Autodesk Inventor part; units mm, degrees
ref_plane "YZ Plane" through (0, 0, 0) normal (1, 0, 0) x (0, 1, 0)
ref_plane "XZ Plane" through (0, 0, 0) normal (0, 1, 0) x (-1, 0, 0)
ref_plane "XY Plane" through (0, 0, 0) normal (0, 0, 1) x (1, 0, 0)
sketch "Sketch1" plane through (0, 0, 0) normal (0, 1, 0) x (-1, 0, 0)
  line L0 (0, 0) -> (48.65, 0)
  line L1 (48.65, 0) -> (48.65, -41.19)
  line L2 (48.65, -41.19) -> (0, -41.19)
  line L3 (0, -41.19) -> (0, 0)
  dimension "d0" = 48.65
  dimension "d1" = 41.19
extrude "Extrusion1" add sketch "Sketch1" along normal blind 1
sketch "Sketch2" plane through (0, 1, 0) normal (0, 1, 0) x (1, 0, 0)
  line L0 (0, 0) -> (-18.8, 0)
  line L1 (-48.65, 0) -> (0, 0)
  line L2 (-18.8, 0) -> (-18.8, 8.64)
  line L3 (0, 0) -> (-33.02, 0)
  line L4 (-30.48, 20.32) -> (-30.48, 21.59)
  line L5 (-30.48, 16.51) -> (-30.48, 13.97)
  line L6 (0, 41.19) -> (-48.65, 41.19)
  line L7 (0, 0) -> (0, 41.19)
  line L8 (-48.65, 41.19) -> (-48.65, 0)
  point P0 (-18.8, 11.18)
  point P1 (-18.8, 13.72)
  point P2 (-18.8, 16.26)
  point P3 (-18.8, 18.8)
  point P4 (-18.8, 21.34)
  point P5 (-18.8, 23.88)
  point P6 (-18.8, 26.42)
  point P7 (-18.8, 28.96)
  point P8 (-18.8, 31.5)
  point P9 (-21.34, 8.64)
  point P10 (-21.34, 11.18)
  point P11 (-21.34, 13.72)
  point P12 (-21.34, 16.26)
  point P13 (-21.34, 18.8)
  point P14 (-21.34, 21.34)
  point P15 (-21.34, 23.88)
  point P16 (-21.34, 26.42)
  point P17 (-21.34, 28.96)
  point P18 (-21.34, 31.5)
  point P19 (-30.48, 24.13)
  point P20 (-46.74, 8.64)
  point P21 (-46.74, 8.64)
  point P22 (-46.74, 11.18)
  point P23 (-46.74, 13.72)
  point P24 (-46.74, 16.26)
  point P25 (-46.74, 18.8)
  point P26 (-46.74, 21.34)
  point P27 (-46.74, 23.88)
  point P28 (-46.74, 26.42)
  point P29 (-46.74, 28.96)
  point P30 (-46.74, 31.5)
  point P31 (-44.2, 8.64)
  point P32 (-44.2, 11.18)
  point P33 (-44.2, 13.72)
  point P34 (-44.2, 16.26)
  point P35 (-44.2, 18.8)
  point P36 (-44.2, 21.34)
  point P37 (-44.2, 23.88)
  point P38 (-44.2, 26.42)
  point P39 (-44.2, 28.96)
  point P40 (-44.2, 31.5)
  point P41 (-30.48, 19.05)
  point P42 (-30.48, 19.05)
  point P43 (-30.48, 24.13)
  point P44 (-30.48, 26.67)
  dimension "d4" = 18.8
  dimension "d5" = 8.64
  dimension "d8" = 2.54
  dimension "d11" = 2.54
  dimension "d14" = 33.02
  dimension "d19" = 2.54
  dimension "d26" = 2.54
  dimension "d77" = 41.19
  dimension "d78" = 48.641
  dimension "d89" = 30.48
hole "Hole1" at (-18.8, 1, -8.64) at (-18.8, 1, -11.18) at (-18.8, 1, -13.72) at (-18.8, 1, -16.26) at (-18.8, 1, -18.8) at (-18.8, 1, -21.34) at (-18.8, 1, -23.88) at (-18.8, 1, -26.42) at (-18.8, 1, -28.96) at (-18.8, 1, -31.5) at (-21.34, 1, -8.64) at (-21.34, 1, -11.18) at (-21.34, 1, -13.72) at (-21.34, 1, -16.26) at (-21.34, 1, -18.8) at (-21.34, 1, -21.34) at (-21.34, 1, -23.88) at (-21.34, 1, -26.42) at (-21.34, 1, -28.96) at (-21.34, 1, -31.5) at (-30.48, 1, -21.59) at (-30.48, 1, -24.13) at (-30.48, 1, -16.51) at (-44.2, 1, -31.5) at (-44.2, 1, -28.96) at (-44.2, 1, -26.42) at (-44.2, 1, -23.88) at (-44.2, 1, -21.34) at (-44.2, 1, -18.8) at (-44.2, 1, -16.26) at (-44.2, 1, -13.72) at (-44.2, 1, -11.18) at (-44.2, 1, -8.64) at (-46.74, 1, -31.5) at (-46.74, 1, -28.96) at (-46.74, 1, -26.42) at (-46.74, 1, -23.88) at (-46.74, 1, -21.34) at (-46.74, 1, -18.8) at (-46.74, 1, -16.26) at (-46.74, 1, -13.72) at (-46.74, 1, -11.18) at (-46.74, 1, -8.64) at (-30.48, 1, -19.05) at (-30.48, 1, -26.67) at (-30.48, 1, -13.97) direction (0, -1, 0) diameter 1.5 end through all
sketch "Sketch3" plane through (0, 1, 0) normal (0, 1, 0) x (1, 0, 0)
  line L0 (-28.956, 38.735) -> (-26.924, 38.735)
  line L1 (-26.924, 38.735) -> (-26.924, 37.465)
  line L2 (-26.924, 37.465) -> (-28.956, 37.465)
  line L3 (-28.956, 37.465) -> (-28.956, 38.735)
  line L4 (-28.956, 38.735) -> (-26.924, 37.465) construction
  line L5 (-26.924, 38.735) -> (-28.956, 37.465) construction
  line L6 (-32.766, 38.735) -> (-30.734, 38.735)
  line L7 (-30.734, 38.735) -> (-30.734, 37.465)
  line L8 (-30.734, 37.465) -> (-32.766, 37.465)
  line L9 (-32.766, 37.465) -> (-32.766, 38.735)
  line L10 (-32.766, 38.735) -> (-30.734, 37.465) construction
  line L11 (-30.734, 38.735) -> (-32.766, 37.465) construction
  line L12 (-36.576, 38.735) -> (-34.544, 38.735)
  line L13 (-34.544, 38.735) -> (-34.544, 37.465)
  line L14 (-34.544, 37.465) -> (-36.576, 37.465)
  line L15 (-36.576, 37.465) -> (-36.576, 38.735)
  line L16 (-36.576, 38.735) -> (-34.544, 37.465) construction
  line L17 (-34.544, 38.735) -> (-36.576, 37.465) construction
  line L18 (-40.386, 38.735) -> (-38.354, 38.735)
  line L19 (-38.354, 38.735) -> (-38.354, 37.465)
  line L20 (-38.354, 37.465) -> (-40.386, 37.465)
  line L21 (-40.386, 37.465) -> (-40.386, 38.735)
  line L22 (-40.386, 38.735) -> (-38.354, 37.465) construction
  line L23 (-38.354, 38.735) -> (-40.386, 37.465) construction
  line L24 (-44.196, 38.735) -> (-42.164, 38.735)
  line L25 (-42.164, 38.735) -> (-42.164, 37.465)
  line L26 (-42.164, 37.465) -> (-44.196, 37.465)
  line L27 (-44.196, 37.465) -> (-44.196, 38.735)
  line L28 (-44.196, 38.735) -> (-42.164, 37.465) construction
  line L29 (-42.164, 38.735) -> (-44.196, 37.465) construction
  line L30 (0, 0) -> (0, 41.19)
  line L31 (-48.65, 0) -> (0, 0)
  point P0 (-27.94, 38.1)
  point P1 (-31.75, 38.1)
  point P2 (-35.56, 38.1)
  point P3 (-39.37, 38.1)
  point P4 (-43.18, 38.1)
  dimension "d40" = 2.032
  dimension "d41" = 1.27
  dimension "d44" = 3.81
  dimension "d88" = 27.94
  dimension "d90" = 38.1
sketch "Sketch4" plane through (0, 1, 0) normal (0, 1, 0) x (1, 0, 0)
  line L0 (-48.65, 0) -> (0, 0)
  line L1 (-3.81, 2.54) -> (-3.81, 5.08)
  line L2 (-3.81, 8.89) -> (-3.81, 11.43)
  line L3 (-3.81, 15.24) -> (-3.81, 17.78)
  line L4 (-3.81, 21.59) -> (-3.81, 24.13)
  line L5 (-3.81, 27.94) -> (-3.81, 30.48)
  point P0 (-3.81, 3.81)
  point P1 (-3.81, 10.16)
  point P2 (-3.81, 16.51)
  point P3 (-3.81, 10.16)
  point P4 (-3.81, 16.51)
  point P5 (-3.81, 16.51)
  point P6 (-3.81, 22.86)
  point P7 (-3.81, 22.86)
  point P8 (-3.81, 22.86)
  point P9 (-3.81, 29.21)
  point P10 (-3.81, 29.21)
  point P11 (-3.81, 29.21)
  dimension "d51" = 3.81
  dimension "d52" = 10.16
  dimension "d53" = 16.51
  dimension "d54" = 1.27
  dimension "d55" = 2.54
  dimension "d58" = 6.35
  dimension "d65" = 6.35
  dimension "d81" = 6.35
hole "Hole2" at (-3.81, 1, -2.54) at (-3.81, 1, -5.08) at (-3.81, 1, -8.89) at (-3.81, 1, -11.43) at (-3.81, 1, -17.78) at (-3.81, 1, -15.24) at (-3.81, 1, -21.59) at (-3.81, 1, -24.13) at (-3.81, 1, -27.94) at (-3.81, 1, -30.48) direction (0, -1, 0) diameter 1.5 end through all
sketch "Sketch5" plane through (0, 1, 0) normal (0, 1, 0) x (1, 0, 0)
  line L0 (-48.65, 0) -> (0, 0)
  line L1 (0, 0) -> (0, 41.19)
  point P0 (-7.239, 25.527)
  point P1 (-18.669, 36.83)
  dimension "d86" = 36.83
  dimension "d87" = 18.669
sketch "Sketch6" plane through (0, 1, 0) normal (0, 1, 0) x (1, 0, 0)
  point P0 (0, 0)
  point P1 (-7.112, 35.814)
properties part number "pcb"
Design review of the part built by this model. Coordinates are the model's own, in mm. Coordinates: 2 decimals unless noted, no trailing zeros. Use CSV: the item, a comma, the result in double quotes. Start each with the question number.
1. To check wall thickness, follow probe 1 along X at (y, z) = (0.65, -31.5); probe 2 along X at (y, z) = (0.2, -29.5); probe 3 along X at (y, z) = (0.7, -13.72). State the ranges of each line that lie inside material, in increasing order.
2. Mouldability with a two-part tool opening along X and no side actions: class faces 1 (the cylindrical face through (-4.035, 0.493, -10.715)), 2 (the flat face through (0, 0.5, -20.9)) as released by +X, released by -X, zero draft, split by the parting line, or undercut.
3. Clearance check with a flat-ended pin moving along its axis: pin 1 (0.9 mm diameter, centred on x = -21.34, z = -18.8, fed in from -Y). State where the tip first meets the part, or that it passes through.
4. Add section A-A on x = -3.81. Count the separate pieces of the cut face and the enclosed holes in it, plus the area to 3 significant figures.
Resolved:
1,probe 1,"-48.65 to -47.49, -45.99 to -44.95, -43.45 to -22.09, -20.59 to -19.55, -18.05 to 0"
1,probe 2,"-48.65 to -47.26, -46.22 to -44.72, -43.68 to -21.86, -20.82 to -19.32, -18.28 to 0"
1,probe 3,"-48.65 to -47.49, -45.99 to -44.95, -43.45 to -31.19, -29.77 to -22.09, -20.59 to -19.55, -18.05 to 0"
2,face 1,"undercut"
2,face 2,"released by +X"
3,pin 1,"through"
4,separate pieces,"11"
4,enclosed holes,"0"
4,area,"26.2 mm2"
